```python
from build123d import *

# Parameters (mm, degrees)
CROQUIS1_W              = 265
CROQUIS1_H              = 110
SALIENTE_EXTRUIR1_DEPTH = 3
CROQUIS2_W              = 3
CROQUIS2_H              = 17.427708433
CORTAR_EXTRUIR1_DEPTH   = 3
CROQUIS4_W              = 259
CROQUIS4_H              = 4
SALIENTE_EXTRUIR3_DEPTH = 3


with BuildPart() as part:
    # Croquis1 → Saliente-Extruir1 (new body)
    with BuildSketch(Plane.XY):
        Rectangle(CROQUIS1_W, CROQUIS1_H)
    extrude(amount=SALIENTE_EXTRUIR1_DEPTH)

    # Croquis2 → Cortar-Extruir1 (cut)
    with BuildSketch(Plane.XY.offset(3)):
        Polygon((-132.5, 55), (-132.5, 37), (-129.5, 37), (-129.5, 52), (-129.5, 55), align=None)
        with Locations((-131, 15.237951406)):
            Rectangle(CROQUIS2_W, CROQUIS2_H)
        Polygon((129.5, 55), (129.5, 52), (129.5, 37), (132.5, 37), (132.5, 55), align=None)
        with Locations((131, 15.237951406)):
            Rectangle(CROQUIS2_W, CROQUIS2_H)
        with Locations((131, -15.237951406)):
            Rectangle(CROQUIS2_W, CROQUIS2_H)
        Polygon((129.5, -37), (129.5, -52), (129.5, -55), (132.5, -55), (132.5, -37), align=None)
        with Locations((-131, -15.237951406)):
            Rectangle(CROQUIS2_W, CROQUIS2_H)
        Polygon((-129.5, -37), (-132.5, -37), (-132.5, -55), (-129.5, -55), (-129.5, -52), align=None)
    extrude(amount=-CORTAR_EXTRUIR1_DEPTH, mode=Mode.SUBTRACT)

    # Croquis4 → Saliente-Extruir3 (add)
    with BuildSketch(Plane(origin=(0, 0, 0), x_dir=(-1, 0, 0), z_dir=(0, 0, -1))):
        with Locations((0, 57)):
            Rectangle(CROQUIS4_W, CROQUIS4_H)
    extrude(amount=-SALIENTE_EXTRUIR3_DEPTH)


solid = part.part
```
CAD build for the part. Positions are in the model's coordinates, mm. Give positions to 0.01 mm unless a question says otherwise; leave off trailing zeros. Loops run counter-clockwise (first coordinate to the right, second up) from the corner with the lowest first, then second, coordinate; pieces in that order, holes last. Notation, with made-up numbers: M 7.5,13.5 L 28.5,13.5 A29 ccw 28.5,41.5 Z; hole C -22,38 d11. An arc over 180 degrees is marked long. Use one line per item in the form item = value.
Item 1: Flat gauge pins, fed straight in: pin 1 (1.5 mm diameter, centred on x = 131.5, z = 1, fed in from +Y); pin 2 (2 mm diameter, centred on x = -15, y = -12, fed in from -Z); pin 3 (0.9 mm diameter, centred on y = 50, z = 1, fed in from -X); pin 4 (1.5 mm diameter, centred on y = 40.5, z = 2, fed in from +X). Where does each tip first touch, or does it go through?
Determined:
pin_1 = 37
pin_2 = 0
pin_3 = -129.5
pin_4 = 129.5
Item 2: Slice it at A-A (y = 48.5). List the corners of the cut face in (x, z).
Determined:
outline = M -129.5,0 L 129.5,0 L 129.5,3 L -129.5,3 Z
Item 3: Drill centre line: probe 1 along X at (y, z) = (17.5, 0.35). Where is it in solid material? Low to high. Write a range as from..to.
Determined:
probe_1 = -129.5..129.5
